The drawing under review shows one solid part. Ordinate dimensions are in mm from its lowest x, y, z. Coordinates: 2 decimals unless noted, no trailing zeros. Write each loop counter-clockwise with the first axis right and the second up, starting at its lowest first coordinate (ties: lowest second). Pieces come first, ordered by that corner, then holes. Notation, with made-up numbers: (36.5, 15) -> (90.5, 15) arc R29 ccw to (90.5, 44) -> close; hole circle Ø3 at (14, -9.5). An arc over 180 degrees is marked (long way). One line per item, written item: value. Start each with the question number.
1) Add section C-C (y = 22.5). State the section outline as (x, z) points, and give its area (3 significant figures).
2) Add section D-D (z = 2.8). State how many separate pieces and enclosed holes the cut face has, and give its area (3 significant figures).
3) Add section A-A (x = 35). State the section outline as (y, z) points, and give its area (3 significant figures).
4) For probe 1 along X at (y, z) = (5, 3.05); probe 2 along Y at (x, z) = (81, 1.15); probe 3 along Y at (x, z) = (79.5, 0.2), list the stretches that pass through material, from the lowest coordinate up. Write a range as from..to.
5) Add section B-B (y = 5). State the section outline as (x, z) points.
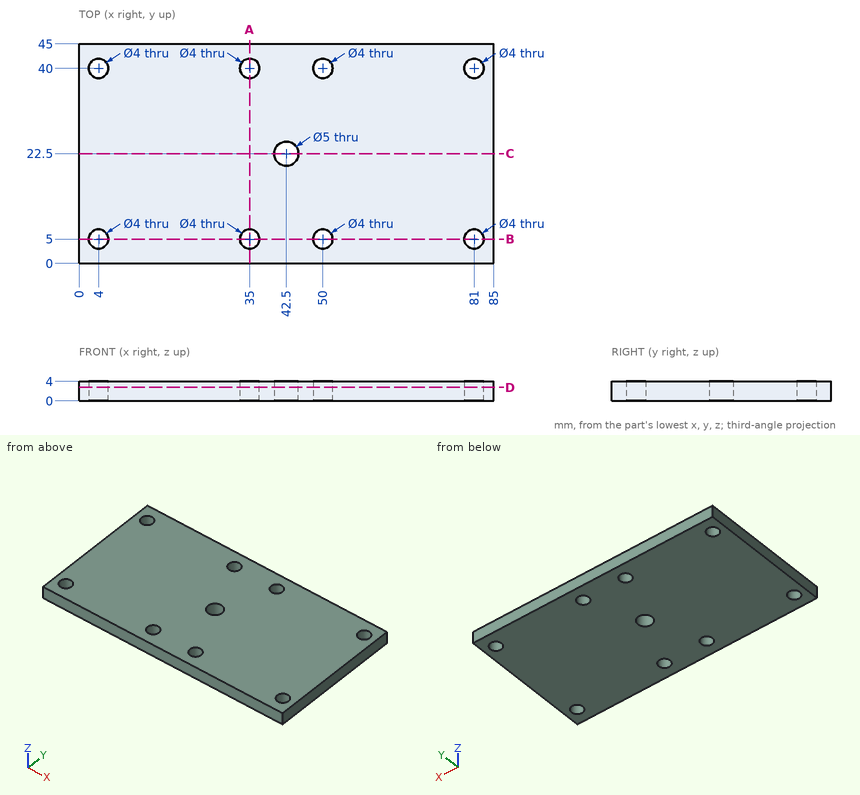
Numbers:
1. outline: (0, 0) -> (40, 0) -> (40, 4) -> (0, 4) -> close; (45, 0) -> (85, 0) -> (85, 4) -> (45, 4) -> close
1. area: 320 mm²
2. separate pieces: 1
2. enclosed holes: 9
2. area: 3,700 mm²
3. outline: (0, 0) -> (3, 0) -> (3, 4) -> (0, 4) -> close; (7, 0) -> (38, 0) -> (38, 4) -> (7, 4) -> close; (42, 0) -> (45, 0) -> (45, 4) -> (42, 4) -> close
3. area: 148 mm²
4. probe 1: 0..2, 6..33, 37..48, 52..79, 83..85
4. probe 2: 0..3, 7..38, 42..45
4. probe 3: 0..3.68, 6.32..38.68, 41.32..45
5. outline: (0, 0) -> (2, 0) -> (2, 4) -> (0, 4) -> close; (6, 0) -> (33, 0) -> (33, 4) -> (6, 4) -> close; (37, 0) -> (48, 0) -> (48, 4) -> (37, 4) -> close; (52, 0) -> (79, 0) -> (79, 4) -> (52, 4) -> close; (83, 0) -> (85, 0) -> (85, 4) -> (83, 4) -> close
